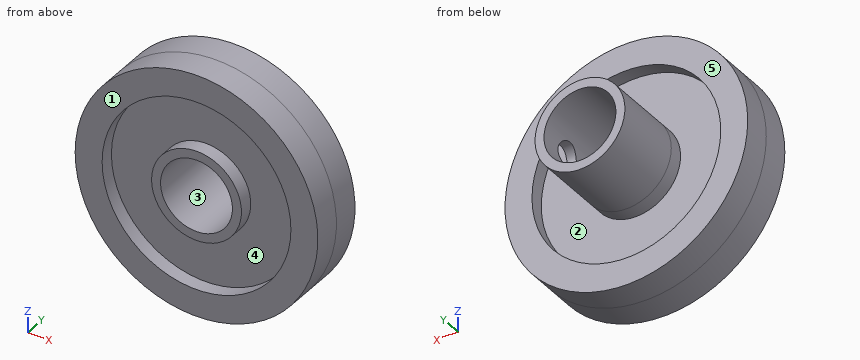
Autodesk Inventor part; units mm, degrees
ref_plane "YZ Plane" through (0, 0, 0) normal (1, 0, 0) x (0, 1, 0)
ref_plane "XZ Plane" through (0, 0, 0) normal (0, 1, 0) x (-1, 0, 0)
ref_plane "XY Plane" through (0, 0, 0) normal (0, 0, 1) x (1, 0, 0)
sketch "Sketch1" plane through (0, 0, 0) normal (0, 1, 0) x (-1, 0, 0)
  circle A0 centre (0, 0) radius 5
  circle A1 centre (0, 0) radius 10.5
  circle A2 centre (0, 0) radius 13.5
  line L0 (0, -18.9) -> (0, 18.9)
  line L1 (-18.9, 0) -> (18.9, 0)
  dimension "d0" = 10
  dimension "d1" = 21
  dimension "d2" = 27
extrude "Extrusion1" add sketch "Sketch1" along normal mid plane 6.35 contours L1 A2 L0 A1 | A1 L0 A2 L1 | A1 L1 A2 L0 | L0 A2 L1 A1
extrude "Extrusion2" add sketch "Sketch1" along normal mid plane 3.175 contours L1 A1 L0 A0 | A0 L0 A1 L1 | A0 L1 A1 L0 | L0 A1 L1 A0
extrude "Extrusion3" add sketch "Sketch1" along normal mid plane 6.35 contours L1 L0 A0 | A0 L0 L1 | L0 L1 A0 | A0 L1 L0
sketch "Sketch2" plane through (0, 3.175, 0) normal (0, 1, 0) x (1, 0, 0)
  circle A0 centre (0, 0) radius 5
extrude "Extrusion4" add sketch "Sketch2" along normal blind 7.9375
sketch "Sketch3" plane through (0, 11.1125, 0) normal (0, 1, 0) x (1, 0, 0)
  circle A0 centre (0, 0) radius 4
  dimension "d11" = 8
extrude "Extrusion5" cut sketch "Sketch3" against normal up to next
sketch "Sketch4" plane through (0, 0, 0) normal (1, 0, 0) x (0, 1, 0)
  circle A0 centre (7.1437, 0) radius 1.5875
  line L0 (11.1125, 4) -> (11.1125, -4)
  line L1 (3.175, 10.5) -> (3.175, -10.5)
  line L2 (3.175, -13.5) -> (3.175, 13.5) construction
  line L3 (3.175, -4) -> (11.1125, -4) construction
  line L4 (11.1125, -4) -> (-3.175, -4) construction
  line L5 (7.1437, -4) -> (7.1437, 4) construction
  line L6 (11.1125, 4) -> (-3.175, 4) construction
  line L7 (-6.0325, 0) -> (13.97, 0) construction
  point P0 (0, 0)
  dimension "d14" = 3.175
extrude "Extrusion6" cut sketch "Sketch4" along normal up to surface
properties part number "Spur Gear" material "Brass, Soft Yellow"
Input: part model. Units: mm. Frame: model coordinates. Face numbers are marked on the shaded views. A direction names the side the tool comes from. Coordinates: 2 decimals unless noted, no trailing zeros. Write each loop counter-clockwise with the first axis right and the second up, starting at its lowest first coordinate (ties: lowest second). Pieces come first, ordered by that corner, then holes.
1) Material intervals for line 1 along X through (y, z) = (2.3, 0); line 2 along Z through (x, y) = (-3.5, -1.75), sorted ascending.
2) Pin query (flat end, axial travel): pin 1 Ø3 at (y, z) = (0, -8) entering from +X; pin 2 Ø1.5 at (x, y) = (-1, 0) entering from -Z; pin 3 Ø13.5 at (x, z) = (-5, -3) entering from +Y; pin 4 Ø3 at (y, z) = (4, -6) entering from +X. Return the tip coordinate at first contact, or that it passes through.
3) Section C-C on y = -2. Output: boundary loops of the cut face in (x, z).
4) Mould query, pull axis X, two halves, no side actions, for the marked faces 1 and 2. Classes: pulls with the +X half, pulls with the -X half, needs draft (parallel to the pull), parting line crosses it, or undercut.
5) Set-up query: the marked faces 3, 4 and 5. Return all of +Z, -Z, +X, -X, +Y, -Y with unobstructed straight access to the full face (end or side cutting, diameter ignored); none if empty.
6) Section A-A on x = 0. Output: boundary loops of the cut face in (y, z) (1 decimal).
7) Section D-D on y = 9.25. Output: boundary loops of the cut face in (x, z), and give its area (3 significant figures).
8) Section B-B on z = 0. Output: boundary loops of the cut face in (x, y) (1 decimal), and give its area (3 significant figures).
Check result:
1. line 1: x = -13.5 to -10.5, -5 to -4, 4 to 5, 10.5 to 13.5
1. line 2: z = -13.04 to -9.9, -3.57 to -1.94, 1.94 to 3.57, 9.9 to 13.04
2. pin 1: stops at x = 11.83
2. pin 2: stops at z = -13.5
2. pin 3: stops at y = 11.11
2. pin 4: stops at x = 12.64
3. outline: circle Ø27 at (0, 0); circle Ø10 at (0, 0); hole circle Ø21 at (0, 0); hole circle Ø8 at (0, 0)
4. face 1: needs draft
4. face 2: undercut
5. face 3: +Y, -Y
5. face 4: -Y
5. face 5: +Y
6. outline: (-3.2, -13.5) - (3.2, -13.5) - (3.2, -10.5) - (1.6, -10.5) - (1.6, -5) - (11.1, -5) - (11.1, -4) - (-3.2, -4) - (-3.2, -5) - (-1.6, -5) - (-1.6, -10.5) - (-3.2, -10.5) - close; (-3.2, 4) - (11.1, 4) - (11.1, 5) - (1.6, 5) - (1.6, 10.5) - (3.2, 10.5) - (3.2, 13.5) - (-3.2, 13.5) - (-3.2, 10.5) - (-1.6, 10.5) - (-1.6, 5) - (-3.2, 5) - close
7. outline: circle Ø10 at (0, 0); hole circle Ø8 at (0, 0)
7. area: 28.3 mm2
8. outline: (-13.5, -3.2) - (-10.5, -3.2) - (-10.5, -1.6) - (-5, -1.6) - (-5, -3.2) - (-4, -3.2) - (-4, 11.1) - (-5, 11.1) - (-5, 1.6) - (-10.5, 1.6) - (-10.5, 3.2) - (-13.5, 3.2) - close; (4, -3.2) - (5, -3.2) - (5, -1.6) - (10.5, -1.6) - (10.5, -3.2) - (13.5, -3.2) - (13.5, 3.2) - (10.5, 3.2) - (10.5, 1.6) - (5, 1.6) - (5, 5.6) - (4, 5.6) - close; (4, 8.7) - (5, 8.7) - (5, 11.1) - (4, 11.1) - close
8. area: 98.4 mm2
